Here's how the part is built. I have some questions about the finished solid (model axes, mm). Face numbers are marked on the shaded views. A direction names the side the tool comes from. Coordinates: 2 decimals unless noted, no trailing zeros. Write each loop counter-clockwise with the first axis right and the second up, starting at its lowest first coordinate (ties: lowest second). Pieces come first, ordered by that corner, then holes.
Item 1: If we mould it in two halves opening along X, with no side actions, what happens to the marked faces 6, 7 and 8? For each: pulls with the +X half, pulls with the -X half, needs draft (parallel to the pull), parting line crosses it, or undercut.
Item 2: I want a section at C-C (x = -5.75). Please give me the cut outline in (y, z).
Item 3: I'm going to push flat-ended pins straight in: P1, Ø2, axis at y = 7.5, z = 4.5, coming from the +X side; P2, Ø6.5, axis at y = -15.5, z = 9, coming from the +X side; P3, Ø1.5, axis at x = -5, z = 4, coming from the -Y side; P4, Ø4, axis at x = -6, y = -27, coming from the +Z side. Where does each tip first touch, or does it pass through?
Item 4: For the marked faces 1, 2, 3, 4 and 5, which set-ups out of +Z, -Z, +X, -X, +Y, -Y let a thin tool reach every point of the face, with its end or its side?
Item 5: Please list where these lines run through material, in increasing order: line 1 (Y direction, x = 0, z = 6.5); line 2 (X direction, y = 0, z = 6.25) (1 decimal); line 3 (X direction, y = -10, z = 11).
Item 6: I want a section at B-B (y = -4). Please give me the cut outline in (x, z).
from build123d import *

# Parameters (mm, degrees)
F1_DEPTH = 12.7
F3_DEPTH = 12.7
F5_DEPTH = 5.08
F6_W     = 5.08
F6_H     = 2.54
F7_DEPTH = 3.175


with BuildPart() as f1:
    # F0 (on Top) → F1 (new body)
    with BuildSketch(Plane.XY):
        with BuildLine():
            Line((-5.08, 6.0989758362), (-5.08, 8.0572467382))
            ThreePointArc((-5.08, 8.0572467382), (0, -9.525), (5.08, 8.0572467382))
            Line((5.08, 8.0572467382), (5.08, 6.0989758362))
            ThreePointArc((5.08, 6.0989758362), (0, -7.9375), (-5.08, 6.0989758362))
        make_face()
    extrude(amount=F1_DEPTH)

    # F2 (on face) → F3 (join, through all)
    with BuildSketch(Plane.XY.offset(12.7)):
        with BuildLine():
            ThreePointArc((2.54, -9.1800885072), (0, -9.525), (-2.54, -9.1800885072))
            Line((-2.54, -9.1800885072), (-2.54, -33.3375))
            Line((-2.54, -33.3375), (2.54, -33.3375))
            Line((2.54, -33.3375), (2.54, -9.1800885072))
        make_face()
    extrude(amount=-F3_DEPTH)

    # F4 (on face) → F5 (cut, through all)
    with BuildSketch(Plane.YZ.offset(2.54)):
        with BuildLine():
            Line((-16.4886742536, 9.525), (-26.0212942536, 9.525))
            ThreePointArc((-26.0212942536, 9.525), (-29.1962942536, 6.35), (-26.0212942536, 3.175))
            Line((-26.0212942536, 3.175), (-16.4886742536, 3.175))
            ThreePointArc((-16.4886742536, 3.175), (-13.3136742536, 6.35), (-16.4886742536, 9.525))
        make_face()
    extrude(amount=-F5_DEPTH, mode=Mode.SUBTRACT)

    # F6 (on face) → F7 (cut, through all)
    with BuildSketch(Plane.XY.offset(12.7)):
        with Locations((0, -21.2587942536)):
            Rectangle(F6_W, F6_H)
    extrude(amount=-F7_DEPTH, mode=Mode.SUBTRACT)


solid = f1.part
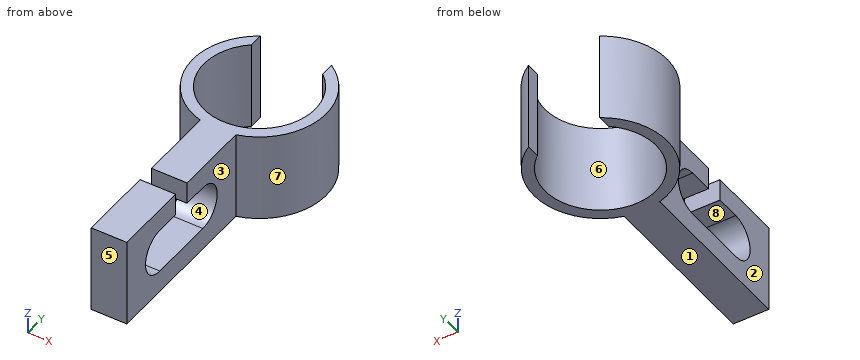
Answer:
1. face 6: undercut
1. face 7: pulls with the +X half
1. face 8: needs draft
2. outline: (-7.59, 0) - (-5.47, 0) - (-5.47, 12.7) - (-7.59, 12.7) - close; (5.47, 0) - (7.59, 0) - (7.59, 12.7) - (5.47, 12.7) - close
3. P1: stops at x = 6.96
3. P2: stops at x = 2.54
3. P3: stops at y = -8.52
3. P4: passes through
4. face 1: -Z, +X, -X, +Y, -Y
4. face 2: +Z, -Z, -X, -Y
4. face 3: +Z, -Z, +X, -Y
4. face 4: +X, -X
4. face 5: +Z, -Z, +X, -X, -Y
5. line 1: y = -33.34 to -29.19, -13.32 to -7.94
5. line 2: x = -9.5 to -7.9, 7.9 to 9.5
5. line 3: x = -2.54 to 2.54
6. outline: (-8.64, 0) - (-6.86, 0) - (-6.86, 12.7) - (-8.64, 12.7) - close; (6.86, 0) - (8.64, 0) - (8.64, 12.7) - (6.86, 12.7) - close
